The listing builds one solid part. Answer for the finished solid, in the listing's coordinates (mm). Round coordinates to 2 decimals unless told otherwise and drop trailing zeros. Loops run counter-clockwise (first coordinate to the right, second up) from the corner with the lowest first, then second, coordinate; pieces in that order, holes last. Notation, with made-up numbers: M 22,-39.75 L 28,-39.75 A23 ccw 28,-29.75 Z; hole C -21,6 d3. An arc over 180 degrees is marked long. Put each result on its own line as item: value. Start each with the question number.
(1) Section C-C, the plane z = 32 is taken. Determine the outline of the cut face in (x, y), then the cut area to 3 significant figures.
(2) Section A-A, the plane x = 72.5 is taken. Determine the outline of the cut face in (y, z).
(3) Straight lines are drawn through the part: line 1 (Z direction, x = -49.45, y = 2.35); line 2 (X direction, y = 2.45, z = 39); line 3 (Z direction, x = -222, y = 2.35). For each, find the intervals that lie inside material, in ascending order.
(4) Flat-ended cylindrical pins translate along their axes: P1, Ø2, axis at y = 2, z = 209.5, coming from the -X side; P2, Ø1.2, axis at x = -145.5, y = 1.5, coming from the +Z side; P3, Ø2, axis at y = 2.5, z = -189.5, coming from the -X side. Find the tip coordinate at first contact, or state that the pin passes through.
(5) Section B-B, the plane y = 1.7 is taken. Count the separate pieces of the cut face and the enclosed holes in it, then the cut area to 3 significant figures.
```python
from build123d import *

# Parameters (mm, degrees)
SKETCH1_W                        = 480
SKETCH1_H                        = 413
BASE_DEPTH                       = 4
SKETCH2_W                        = 20
SKETCH2_H                        = 5
TOP_TABS_DEFINITION_DEPTH        = 4
TOP_TABS_PATTERN_COUNT           = 5
TOP_TABS_PATTERN_PITCH           = 55
TOP_TABS_PATTERN_COL_COUNT       = 5
TOP_TABS_PATTERN_COL_PITCH       = 55
BOTTOM_TABS_COPY_1_SKETCH_W      = 20
BOTTOM_TABS_COPY_1_SKETCH_H      = 5
BOTTOM_TABS_COPY_1_DEPTH         = 4
BOTTOM_TABS_COPY_2_SKETCH_W      = 20
BOTTOM_TABS_COPY_2_SKETCH_H      = 5
BOTTOM_TABS_COPY_2_DEPTH         = 4
BOTTOM_TABS_COPY_3_SKETCH_W      = 20
BOTTOM_TABS_COPY_3_SKETCH_H      = 5
BOTTOM_TABS_COPY_3_DEPTH         = 4
BOTTOM_TABS_COPY_4_SKETCH_W      = 20
BOTTOM_TABS_COPY_4_SKETCH_H      = 5
BOTTOM_TABS_COPY_4_DEPTH         = 4
BOTTOM_TABS_COPY_5_SKETCH_W      = 20
BOTTOM_TABS_COPY_5_SKETCH_H      = 5
BOTTOM_TABS_COPY_5_DEPTH         = 4
BOTTOM_TABS_COPY_6_SKETCH_W      = 20
BOTTOM_TABS_COPY_6_SKETCH_H      = 5
BOTTOM_TABS_COPY_6_DEPTH         = 4
BOTTOM_TABS_COPY_7_SKETCH_W      = 20
BOTTOM_TABS_COPY_7_SKETCH_H      = 5
BOTTOM_TABS_COPY_7_DEPTH         = 4
BOTTOM_TABS_COPY_8_SKETCH_W      = 20
BOTTOM_TABS_COPY_8_SKETCH_H      = 5
BOTTOM_TABS_COPY_8_DEPTH         = 4
ELECTRONICS_MOUNTING_HOLES_1_5_D = 1.5
SKETCH7_W                        = 5
SKETCH7_H                        = 20
LEFT_TABS_DEFINITION_DEPTH       = 4
LEFT_TABS_PATTERN_COUNT          = 4
LEFT_TABS_PATTERN_PITCH          = 55
LEFT_TABS_PATTERN_COL_COUNT      = 4
LEFT_TABS_PATTERN_COL_PITCH      = 55
RIGHT_TABS_COPY_1_SKETCH_W       = 5
RIGHT_TABS_COPY_1_SKETCH_H       = 20
RIGHT_TABS_COPY_1_DEPTH          = 4
RIGHT_TABS_COPY_2_SKETCH_W       = 5
RIGHT_TABS_COPY_2_SKETCH_H       = 20
RIGHT_TABS_COPY_2_DEPTH          = 4
RIGHT_TABS_COPY_3_SKETCH_W       = 5
RIGHT_TABS_COPY_3_SKETCH_H       = 20
RIGHT_TABS_COPY_3_DEPTH          = 4
RIGHT_TABS_COPY_4_SKETCH_W       = 5
RIGHT_TABS_COPY_4_SKETCH_H       = 20
RIGHT_TABS_COPY_4_DEPTH          = 4
RIGHT_TABS_COPY_5_SKETCH_W       = 5
RIGHT_TABS_COPY_5_SKETCH_H       = 20
RIGHT_TABS_COPY_5_DEPTH          = 4
RIGHT_TABS_COPY_6_SKETCH_W       = 5
RIGHT_TABS_COPY_6_SKETCH_H       = 20
RIGHT_TABS_COPY_6_DEPTH          = 4
M6_CLEARANCE_HOLE1_D             = 5
TAP_DRILL_FOR_M3X0_5_TAP1_D      = 2.5


with BuildPart() as part:
    # Sketch1 → Base (new body)
    with BuildSketch(Plane(origin=(0, 0, 0), x_dir=(1, 0, 0), z_dir=(0, 1, 0))):
        Rectangle(SKETCH1_W, SKETCH1_H)
    extrude(amount=BASE_DEPTH)

    # Sketch2 → Top Tabs Definition (add)
    with BuildSketch(Plane(origin=(0, 4, 0), x_dir=(1, 0, 0), z_dir=(0, 1, 0))):
        with Locations((0, 209)):
            Rectangle(SKETCH2_W, SKETCH2_H)
    top_tabs_definition = extrude(amount=-TOP_TABS_DEFINITION_DEPTH)

    # Top Tabs Pattern: Top Tabs Definition ×5
    with Locations(*[(-i * TOP_TABS_PATTERN_PITCH, 0, 0) for i in range(1, TOP_TABS_PATTERN_COUNT)]):
        add(top_tabs_definition)

    # Top Tabs Pattern col: Top Tabs Definition ×5
    with Locations(*[(i * TOP_TABS_PATTERN_COL_PITCH, 0, 0) for i in range(1, TOP_TABS_PATTERN_COL_COUNT)]):
        add(top_tabs_definition)

    # Bottom Tabs: Top Tabs Definition across plane
    add(top_tabs_definition.mirror(Plane.XY))

    # Bottom Tabs copy 1 sketch → Bottom Tabs copy 1 (add)
    with BuildSketch(Plane(origin=(-55, 4, 0), x_dir=(1, 0, 0), z_dir=(0, 1, 0))):
        with Locations((0, -209)):
            Rectangle(BOTTOM_TABS_COPY_1_SKETCH_W, BOTTOM_TABS_COPY_1_SKETCH_H)
    extrude(amount=-BOTTOM_TABS_COPY_1_DEPTH)

    # Bottom Tabs copy 2 sketch → Bottom Tabs copy 2 (add)
    with BuildSketch(Plane(origin=(-110, 4, 0), x_dir=(1, 0, 0), z_dir=(0, 1, 0))):
        with Locations((0, -209)):
            Rectangle(BOTTOM_TABS_COPY_2_SKETCH_W, BOTTOM_TABS_COPY_2_SKETCH_H)
    extrude(amount=-BOTTOM_TABS_COPY_2_DEPTH)

    # Bottom Tabs copy 3 sketch → Bottom Tabs copy 3 (add)
    with BuildSketch(Plane(origin=(-165, 4, 0), x_dir=(1, 0, 0), z_dir=(0, 1, 0))):
        with Locations((0, -209)):
            Rectangle(BOTTOM_TABS_COPY_3_SKETCH_W, BOTTOM_TABS_COPY_3_SKETCH_H)
    extrude(amount=-BOTTOM_TABS_COPY_3_DEPTH)

    # Bottom Tabs copy 4 sketch → Bottom Tabs copy 4 (add)
    with BuildSketch(Plane(origin=(-220, 4, 0), x_dir=(1, 0, 0), z_dir=(0, 1, 0))):
        with Locations((0, -209)):
            Rectangle(BOTTOM_TABS_COPY_4_SKETCH_W, BOTTOM_TABS_COPY_4_SKETCH_H)
    extrude(amount=-BOTTOM_TABS_COPY_4_DEPTH)

    # Bottom Tabs copy 5 sketch → Bottom Tabs copy 5 (add)
    with BuildSketch(Plane(origin=(55, 4, 0), x_dir=(1, 0, 0), z_dir=(0, 1, 0))):
        with Locations((0, -209)):
            Rectangle(BOTTOM_TABS_COPY_5_SKETCH_W, BOTTOM_TABS_COPY_5_SKETCH_H)
    extrude(amount=-BOTTOM_TABS_COPY_5_DEPTH)

    # Bottom Tabs copy 6 sketch → Bottom Tabs copy 6 (add)
    with BuildSketch(Plane(origin=(110, 4, 0), x_dir=(1, 0, 0), z_dir=(0, 1, 0))):
        with Locations((0, -209)):
            Rectangle(BOTTOM_TABS_COPY_6_SKETCH_W, BOTTOM_TABS_COPY_6_SKETCH_H)
    extrude(amount=-BOTTOM_TABS_COPY_6_DEPTH)

    # Bottom Tabs copy 7 sketch → Bottom Tabs copy 7 (add)
    with BuildSketch(Plane(origin=(165, 4, 0), x_dir=(1, 0, 0), z_dir=(0, 1, 0))):
        with Locations((0, -209)):
            Rectangle(BOTTOM_TABS_COPY_7_SKETCH_W, BOTTOM_TABS_COPY_7_SKETCH_H)
    extrude(amount=-BOTTOM_TABS_COPY_7_DEPTH)

    # Bottom Tabs copy 8 sketch → Bottom Tabs copy 8 (add)
    with BuildSketch(Plane(origin=(220, 4, 0), x_dir=(1, 0, 0), z_dir=(0, 1, 0))):
        with Locations((0, -209)):
            Rectangle(BOTTOM_TABS_COPY_8_SKETCH_W, BOTTOM_TABS_COPY_8_SKETCH_H)
    extrude(amount=-BOTTOM_TABS_COPY_8_DEPTH)

    # Electronics Mounting Holes (1.5) (through all)
    with Locations(Plane(origin=(0, 4, 0), x_dir=(1, 0, 0), z_dir=(0, 1, 0))):
        with Locations((-49.45, 143.854151385), (-49.45, 101.854151385), (41.55, 110.854151385), (59.05, 144.354151385), (90.05, 144.354151385), (90.05, 91.354151385), (59.05, 91.354151385), (161.815, 95.130848615), (161.815, 53.220848615), (161.815, 155.130848615), (161.815, 113.220848615), (227.855, 110.045848615), (227.855, 158.305848615), (227.855, 50.045848615), (227.855, 98.305848615), (-162.5, 28.854151385), (-162.5, 89.854151385), (-223.5, 89.854151385), (-223.5, 28.854151385)):
            Hole(ELECTRONICS_MOUNTING_HOLES_1_5_D / 2)

    # Sketch7 → Left Tabs Definition (add)
    with BuildSketch(Plane(origin=(0, 4, 0), x_dir=(1, 0, 0), z_dir=(0, 1, 0))):
        with Locations((-242.5, 0)):
            Rectangle(SKETCH7_W, SKETCH7_H)
    left_tabs_definition = extrude(amount=-LEFT_TABS_DEFINITION_DEPTH)

    # Left Tabs Pattern: Left Tabs Definition ×4
    with Locations(*[(0, 0, -i * LEFT_TABS_PATTERN_PITCH) for i in range(1, LEFT_TABS_PATTERN_COUNT)]):
        add(left_tabs_definition)

    # Left Tabs Pattern col: Left Tabs Definition ×4
    with Locations(*[(0, 0, i * LEFT_TABS_PATTERN_COL_PITCH) for i in range(1, LEFT_TABS_PATTERN_COL_COUNT)]):
        add(left_tabs_definition)

    # Right Tabs: Left Tabs Definition across plane
    add(left_tabs_definition.mirror(Plane(origin=(0, 0, 0), x_dir=(0, 0, 1), z_dir=(1, 0, 0))))

    # Right Tabs copy 1 sketch → Right Tabs copy 1 (add)
    with BuildSketch(Plane(origin=(0, 4, -55), x_dir=(-1, 0, 0), z_dir=(0, 1, 0))):
        with Locations((-242.5, 0)):
            Rectangle(RIGHT_TABS_COPY_1_SKETCH_W, RIGHT_TABS_COPY_1_SKETCH_H)
    extrude(amount=-RIGHT_TABS_COPY_1_DEPTH)

    # Right Tabs copy 2 sketch → Right Tabs copy 2 (add)
    with BuildSketch(Plane(origin=(0, 4, -110), x_dir=(-1, 0, 0), z_dir=(0, 1, 0))):
        with Locations((-242.5, 0)):
            Rectangle(RIGHT_TABS_COPY_2_SKETCH_W, RIGHT_TABS_COPY_2_SKETCH_H)
    extrude(amount=-RIGHT_TABS_COPY_2_DEPTH)

    # Right Tabs copy 3 sketch → Right Tabs copy 3 (add)
    with BuildSketch(Plane(origin=(0, 4, -165), x_dir=(-1, 0, 0), z_dir=(0, 1, 0))):
        with Locations((-242.5, 0)):
            Rectangle(RIGHT_TABS_COPY_3_SKETCH_W, RIGHT_TABS_COPY_3_SKETCH_H)
    extrude(amount=-RIGHT_TABS_COPY_3_DEPTH)

    # Right Tabs copy 4 sketch → Right Tabs copy 4 (add)
    with BuildSketch(Plane(origin=(0, 4, 55), x_dir=(-1, 0, 0), z_dir=(0, 1, 0))):
        with Locations((-242.5, 0)):
            Rectangle(RIGHT_TABS_COPY_4_SKETCH_W, RIGHT_TABS_COPY_4_SKETCH_H)
    extrude(amount=-RIGHT_TABS_COPY_4_DEPTH)

    # Right Tabs copy 5 sketch → Right Tabs copy 5 (add)
    with BuildSketch(Plane(origin=(0, 4, 110), x_dir=(-1, 0, 0), z_dir=(0, 1, 0))):
        with Locations((-242.5, 0)):
            Rectangle(RIGHT_TABS_COPY_5_SKETCH_W, RIGHT_TABS_COPY_5_SKETCH_H)
    extrude(amount=-RIGHT_TABS_COPY_5_DEPTH)

    # Right Tabs copy 6 sketch → Right Tabs copy 6 (add)
    with BuildSketch(Plane(origin=(0, 4, 165), x_dir=(-1, 0, 0), z_dir=(0, 1, 0))):
        with Locations((-242.5, 0)):
            Rectangle(RIGHT_TABS_COPY_6_SKETCH_W, RIGHT_TABS_COPY_6_SKETCH_H)
    extrude(amount=-RIGHT_TABS_COPY_6_DEPTH)

    # M6 Clearance Hole1 (through all)
    with Locations(Plane(origin=(0, 4, 0), x_dir=(1, 0, 0), z_dir=(0, 1, 0))):
        with Locations((-147.5, -40.969284902), (-22.5, -40.969284902), (102.5, -40.969284902)):
            Hole(M6_CLEARANCE_HOLE1_D / 2)

    # Tap Drill for M3x0.5 Tap1 (through all)
    with Locations(Plane(origin=(0, 0, 0), x_dir=(-1, 0, 0), z_dir=(0, -1, 0))):
        with Locations((120, 122.854151385), (222, 142.854151385)):
            Hole(TAP_DRILL_FOR_M3X0_5_TAP1_D / 2)


solid = part.part
```
Recorded:
1. outline: M -240,0 L 240,0 L 240,4 L -240,4 Z
1. area: 1,920 mm²
2. outline: M 0,-206.5 L 4,-206.5 L 4,206.5 L 0,206.5 Z
3. line 1: z = -211.5 to -144.6, -143.1 to -102.6, -101.1 to 211.5
3. line 2: x = -240 to -149.04, -145.96 to -24.04, -20.96 to 100.96, 104.04 to 240
3. line 3: z = -211.5 to -144.1, -141.6 to 211.5
4. P1: stops at x = -230
4. P2: stops at z = 206.5
4. P3: stops at x = -240
5. separate pieces: 1
5. enclosed holes: 24
5. area: 201,000 mm²
